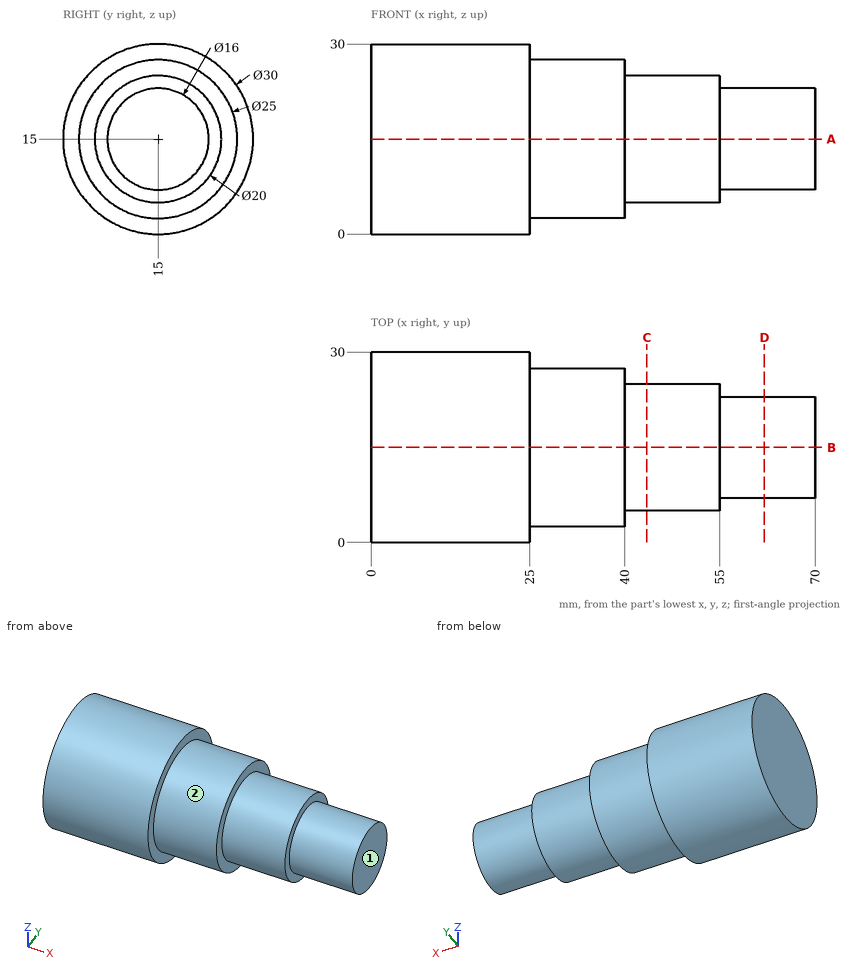
Job drawing, mm, ordinate dimensions from the low corner. One solid piece. A direction names the side the tool comes from. Round coordinates to 2 decimals unless told otherwise and drop trailing zeros. Loops run counter-clockwise (first coordinate to the right, second up) from the corner with the lowest first, then second, coordinate; pieces in that order, holes last. Notation, with made-up numbers: (-40, 76.25) -> (-1, 76.25) arc R37 ccw to (-1, 112.25) -> close; hole circle Ø2 at (88.25, 86). An arc over 180 degrees is marked (long way). Use a Markdown table: item, result.
1) Tool access for the marked faces 1 and 2: list every direction of +Z, -Z, +X, -X, +Y, -Y with a clear straight run to the whole face (end or side of a thin tool).
The answers:
| item | result |
|---|---|
| face 1 | +Z, -Z, +X, +Y, -Y |
| face 2 | +X |
2) Cut at A-A, the plane z = 15. List the corners of the cut face in (x, y).
The answers:
| item | result |
|---|---|
| outline | (0, 0) -> (25, 0) -> (25, 2.5) -> (40, 2.5) -> (40, 5) -> (55, 5) -> (55, 7) -> (70, 7) -> (70, 23) -> (55, 23) -> (55, 25) -> (40, 25) -> (40, 27.5) -> (25, 27.5) -> (25, 30) -> (0, 30) -> close |
3) Cut at D-D, the plane x = 62. List the corners of the cut face in (y, z), and give its area (3 significant figures).
The answers:
| item | result |
|---|---|
| outline | circle Ø16 at (15, 15) |
| area | 201 mm2 |
4) Drop flat-ended pins along their axis: pin 1 Ø8 at (x, y) = (7.5, 22) entering from +Z; pin 2 Ø6 at (x, y) = (15.5, 6.5) entering from -Z; pin 3 Ø8 at (x, y) = (17, 20.5) entering from +Z. Give the stop position or say it passes through.
The answers:
| item | result |
|---|---|
| pin 1 | stops at z = 29.7 |
| pin 2 | stops at z = 1.04 |
| pin 3 | stops at z = 29.92 |
5) Cut at C-C, the plane x = 43.5. List the corners of the cut face in (y, z).
The answers:
| item | result |
|---|---|
| outline | circle Ø20 at (15, 15) |
6) Probe line 1 (X direction, y = 19.25, z = 6.5); line 2 (X direction, y = 27.75, z = 9.5); line 3 (Z direction, x = 22, y = 11). List the from-to ranges inside material, lowest first. Write a range as [from, to].
The answers:
| item | result |
|---|---|
| line 1 | x = [0, 55] |
| line 2 | x = [0, 25] |
| line 3 | z = [0.54, 29.46] |
